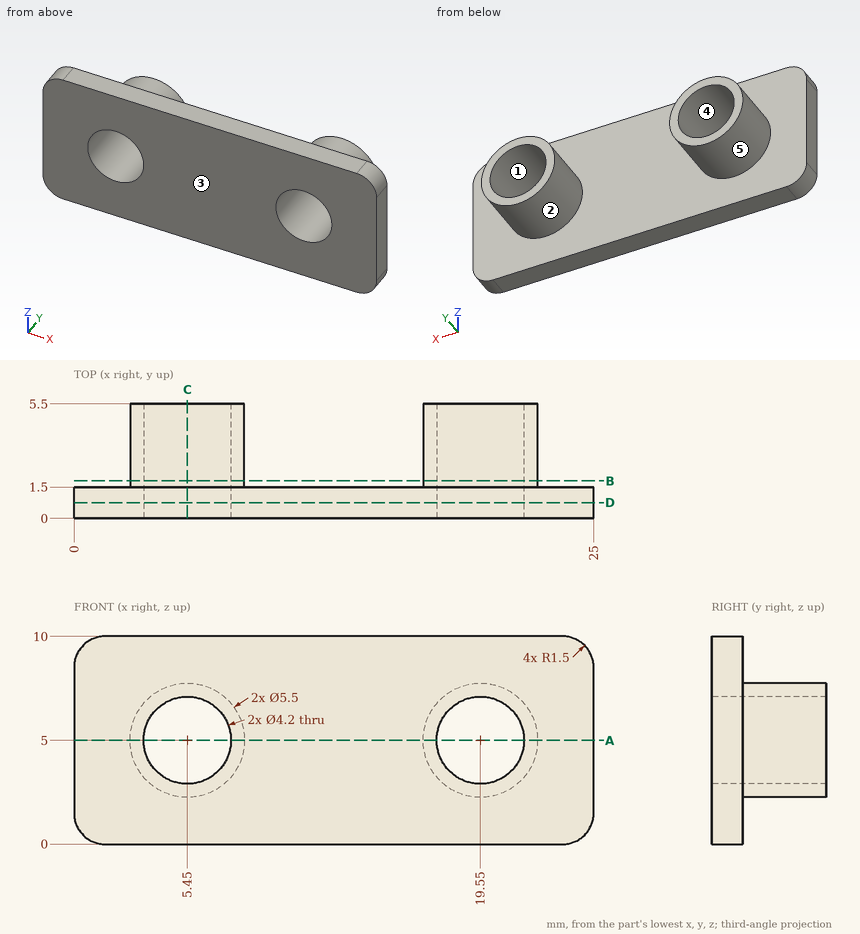
Study the drawing (mm; zero at the part's minimum x, y, z) and answer. A direction names the side the tool comes from. Give positions to 0.01 mm unless a question says otherwise; leave off trailing zeros. Order: outer loops, then holes, each group sorted by start corner. A loop starts at its lowest first (then second) coordinate and runs counter-clockwise, first axis right, second up. Notation, with made-up numbers: (36.25, 45) - (89.25, 45) arc R24 cw to (89.25, 81) - close; hole circle Ø9 at (40, -35.5). An arc over 180 degrees is marked (long way). Answer as CSV lines item,"result". Start each with the question number.
Q1. The part is cut by section C-C (x = 5.45). Write down the section's boundary in (y, z), then the cut area to 3 significant figures.
Q2. For the marked faces 4 and 5, determine the directions among +Z, -Z, +X, -X, +Y, -Y from which every point of the face is accessible in a straight line to the end or side of a thin tool.
Q3. Find the intervals of material crossed by L1, parallel to X at y = 1.45, z = 6.75; L2, parallel to Z at x = 19.55, y = 2.7; L3, parallel to X at y = 1.45, z = 3.75, in increasing order. Write a range as [from, to].
Q4. The part is cut by section D-D (y = 0.75). Write down the section's boundary in (x, z).
Q5. The mould has two halves that part along Z. Classify the marked faces 1, 2 and 3: +Z half, -Z half, draft (parallel to the pull), parting line (faces both ways), or undercut.
Q6. Given pin 1 Ø3 at (x, y) = (5, 4) entering from +Z, flat-ended and moving along its own axis, determine where the tip first touches the part or whether it passes through.
Q7. The part is cut by section A-A (z = 5). Write down the section's boundary in (x, y), then the cut area to 3 significant figures.
Q8. The part is cut by section B-B (y = 1.8). Write down the section's boundary in (x, z), then the cut area to 3 significant figures.
Check result:
1,outline,"(0, 0) - (1.5, 0) - (1.5, 2.25) - (5.5, 2.25) - (5.5, 2.9) - (0, 2.9) - close; (0, 7.1) - (5.5, 7.1) - (5.5, 7.75) - (1.5, 7.75) - (1.5, 10) - (0, 10) - close"
1,area,"13.9 mm²"
2,face 4,"+Y, -Y"
2,face 5,"+Y"
3,L1,"x = [0, 4.29], [6.61, 18.39], [20.71, 25]"
3,L2,"z = [2.25, 2.9], [7.1, 7.75]"
3,L3,"x = [0, 3.76], [7.14, 17.86], [21.24, 25]"
4,outline,"(0, 1.5) arc R1.5 ccw to (1.5, 0) - (23.5, 0) arc R1.5 ccw to (25, 1.5) - (25, 8.5) arc R1.5 ccw to (23.5, 10) - (1.5, 10) arc R1.5 ccw to (0, 8.5) - close; hole circle Ø4.2 at (5.45, 5); hole circle Ø4.2 at (19.55, 5)"
5,face 1,"undercut"
5,face 2,"parting line"
5,face 3,"draft"
6,pin 1,"stops at z = 7.75"
7,outline,"(0, 0) - (3.35, 0) - (3.35, 5.5) - (2.7, 5.5) - (2.7, 1.5) - (0, 1.5) - close; (7.55, 0) - (17.45, 0) - (17.45, 5.5) - (16.8, 5.5) - (16.8, 1.5) - (8.2, 1.5) - (8.2, 5.5) - (7.55, 5.5) - close; (21.65, 0) - (25, 0) - (25, 1.5) - (22.3, 1.5) - (22.3, 5.5) - (21.65, 5.5) - close"
7,area,"35.3 mm²"
8,outline,"circle Ø5.5 at (5.45, 5); circle Ø5.5 at (19.55, 5); hole circle Ø4.2 at (5.45, 5); hole circle Ø4.2 at (19.55, 5)"
8,area,"19.8 mm²"
